from build123d import *

# Parameters (mm, degrees)
SKETCH1_R           = 2.5527
BOSS_EXTRUDE1_DEPTH = 6.35
CUT_EXTRUDE1_DEPTH  = 85.78424365


with BuildPart() as part:
    # Sketch1 → Boss-Extrude1 (new body)
    with BuildSketch(Plane.XY):
        with BuildLine():
            Line((1.487897552, 1.487897552), (41.309178157, 41.309178157))
            ThreePointArc((41.309178157, 41.309178157), (44.901280605, 42.797075708), (48.493383054, 41.309178157))
            Line((48.493383054, 41.309178157), (66.094685051, 23.70787616))
            ThreePointArc((66.094685051, 23.70787616), (67.582582603, 20.115773711), (66.094685051, 16.523671263))
            Line((66.094685051, 16.523671263), (0.25891134, -49.312102448))
            ThreePointArc((0.25891134, -49.312102448), (-1.389159272, -50.413308025), (-3.333191109, -50.8))
            Line((-3.333191109, -50.8), (-58.42, -50.8))
            ThreePointArc((-58.42, -50.8), (-62.012102448, -49.312102448), (-63.5, -45.72))
            Line((-63.5, -45.72), (-63.5, -5.08))
            ThreePointArc((-63.5, -5.08), (-62.012102448, -1.487897552), (-58.42, 0))
            Line((-58.42, 0), (-2.104204897, 0))
            ThreePointArc((-2.104204897, 0), (-0.16017306, 0.386691975), (1.487897552, 1.487897552))
        make_face()
        with Locations((-50.8, -12.7)):
            Circle(SKETCH1_R, mode=Mode.SUBTRACT)
        with Locations((-25.4, -12.7)):
            Circle(SKETCH1_R, mode=Mode.SUBTRACT)
        with Locations((-25.4, -38.1)):
            Circle(SKETCH1_R, mode=Mode.SUBTRACT)
        with Locations((-50.8, -38.1)):
            Circle(SKETCH1_R, mode=Mode.SUBTRACT)
    extrude(amount=BOSS_EXTRUDE1_DEPTH)

    # Sketch2 → Cut-Extrude1 (cut, through all)
    with BuildSketch(Plane.XY.offset(6.35)):
        with BuildLine():
            Line((-2.104204897, 0), (-17.78, 0))
            ThreePointArc((-17.78, 0), (-14.187897552, -1.487897552), (-12.7, -5.08))
            Line((-12.7, -5.08), (-12.7, -45.72))
            ThreePointArc((-12.7, -45.72), (-14.187897552, -49.312102448), (-17.78, -50.8))
            Line((-17.78, -50.8), (-3.333191109, -50.8))
            ThreePointArc((-3.333191109, -50.8), (-1.389159272, -50.413308025), (0.25891134, -49.312102448))
            Line((0.25891134, -49.312102448), (66.094685051, 16.523671263))
            ThreePointArc((66.094685051, 16.523671263), (67.582582603, 20.115773711), (66.094685051, 23.70787616))
            Line((66.094685051, 23.70787616), (48.493383054, 41.309178157))
            ThreePointArc((48.493383054, 41.309178157), (44.901280605, 42.797075708), (41.309178157, 41.309178157))
            Line((41.309178157, 41.309178157), (1.487897552, 1.487897552))
            ThreePointArc((1.487897552, 1.487897552), (-0.16017306, 0.386691975), (-2.104204897, 0))
        make_face()
    extrude(amount=-CUT_EXTRUDE1_DEPTH, mode=Mode.SUBTRACT)


solid = part.part
Source: CAD feature listing. Evaluate the final solid. Frame: model axes, mm. Give positions to 0.01 mm unless a question says otherwise; leave off trailing zeros. Order: outer loops, then holes, each group sorted by start corner. A loop starts at its lowest first (then second) coordinate and runs counter-clockwise, first axis right, second up. Notation, with made-up numbers: (49, 39) -> (85, 39) arc R14 ccw to (85, 53) -> close; hole circle Ø6 at (57.25, 36). An arc over 180 degrees is marked (long way). Write item = value, one per line.
Q1. Cut plane B-B, the plane y = -12.7. Output: boundary loops of the cut face in (x, z).
Data:
outline = (-63.5, 0) -> (-53.35, 0) -> (-53.35, 6.35) -> (-63.5, 6.35) -> close; (-48.25, 0) -> (-27.95, 0) -> (-27.95, 6.35) -> (-48.25, 6.35) -> close; (-22.85, 0) -> (-12.7, 0) -> (-12.7, 6.35) -> (-22.85, 6.35) -> close
Q2. Cut plane C-C, the plane z = 4. Output: boundary loops of the cut face in (x, y), and give its area (3 significant figures).
Data:
outline = (-63.5, -45.72) arc R5.08 ccw to (-58.42, -50.8) -> (-17.78, -50.8) arc R5.08 ccw to (-12.7, -45.72) -> (-12.7, -5.08) arc R5.08 ccw to (-17.78, 0) -> (-58.42, 0) arc R5.08 ccw to (-63.5, -5.08) -> close; hole circle Ø5.11 at (-50.8, -38.1); hole circle Ø5.11 at (-50.8, -12.7); hole circle Ø5.11 at (-25.4, -38.1); hole circle Ø5.11 at (-25.4, -12.7)
area = 2,480 mm^2
Q3. Material intervals for line 1 (Y direction, x = -50.8, z = 3.5); line 2 (Y direction, x = -49, z = 0.5); line 3 (X direction, y = -5, z = 4.5), sorted ascending. Write a range as from..to.
Data:
line_1 = -50.8..-40.65, -35.55..-15.25, -10.15..0
line_2 = -50.8..-39.91, -36.29..-14.51, -10.89..0
line_3 = -63.5..-12.7
Q4. Pin query (flat end, axial travel): pin 1 (10 mm diameter, centred on x = -39.5, y = -28.5, fed in from -Z); pin 2 (4 mm diameter, centred on x = -50.8, y = -12.7, fed in from -Z). Return the tip coordinate at first contact, or that it passes through.
Data:
pin_1 = 0
pin_2 = through
Q5. Cut plane A-A, the plane x = -25.4. Output: boundary loops of the cut face in (y, z).
Data:
outline = (-50.8, 0) -> (-40.65, 0) -> (-40.65, 6.35) -> (-50.8, 6.35) -> close; (-35.55, 0) -> (-15.25, 0) -> (-15.25, 6.35) -> (-35.55, 6.35) -> close; (-10.15, 0) -> (0, 0) -> (0, 6.35) -> (-10.15, 6.35) -> close
Q6. Pull-direction query (X, two-part tool) for faces 1 (the face through (-48.365, -11.933, 3.131)), 2 (the face through (-38, -25, 0)), 3 (the face through (-14.228, -1.449, 3.219)), 4 (the face through (-27.281, -36.375, 3.131)); classes: released by +X, released by -X, zero draft, split by the parting line, or undercut.
Data:
face_1 = undercut
face_2 = zero draft
face_3 = released by +X
face_4 = undercut
